Check sheet for the modelled part. Datum: model origin and axes. Units: mm. Face numbers are marked on the shaded views. A direction names the side the tool comes from. Round coordinates to 2 decimals unless told otherwise and drop trailing zeros. Loops run counter-clockwise (first coordinate to the right, second up) from the corner with the lowest first, then second, coordinate; pieces in that order, holes last. Notation, with made-up numbers: (81.25, -8.5) - (125.25, -8.5) arc R21 cw to (125.25, 19.5) - close; hole circle Ø8 at (13.25, 35.5). An arc over 180 degrees is marked (long way). Answer in a Markdown table with one row per item. Add a question column.
(1) Access from +Z, -Z, +X, -X, +Y, -Y to the whole of each face (thin tool, end or side, straight path). Record for the marked faces 1, 2, 3 and 4.
(2) Thickness scan on line 1 along Y through (x, z) = (0, 3.75); line 2 along Y through (x, z) = (2.5, 1.6); line 3 along Y through (x, z) = (-3, 2.25). Record the ranges inside material, lowest first.
(3) Gauge pin test, flat ends, axial feed: pin 1 (1.9 mm diameter, centred on x = 0, y = -8, fed in from -Z); pin 2 (1.8 mm diameter, centred on x = 1, y = -6.5, fed in from -Z); pin 3 (2.5 mm diameter, centred on x = 3.5, y = 0, fed in from +Z). Record the tip position at first contact, or that the pin passes through.
(4) Cross-section at A-A on z = 4.65. Enter the section's corners in (x, y).
(5) Cross-section at C-C on z = 3.1. Enter the section's corners in (x, y).
(6) Mould release check, pull along X, two halves, no side actions. Record for the marked faces 5, 6 and 7: +X half, -X half, draft (parallel to the pull), parting line (faces both ways), or undercut.
(7) Cross-section at B-B on x = 0. Enter the section's corners in (y, z), then the cut area to 3 significant figures.
(8) Cross-section at D-D on y = 0.5. Enter the section's corners in (x, z).
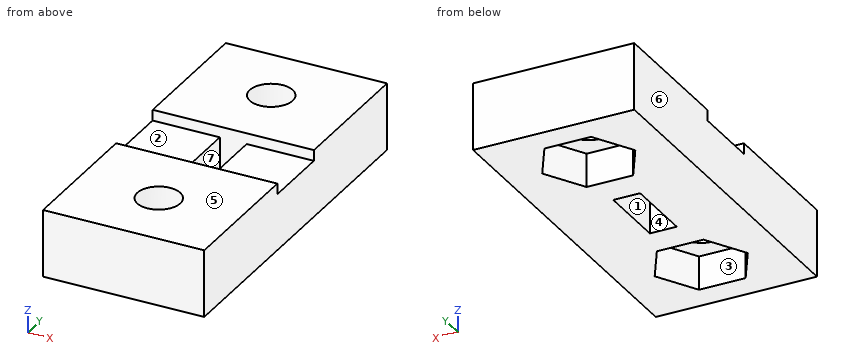
from build123d import *

# Parameters (mm, degrees)
SKETCH1_W           = 12
SKETCH1_H           = 26
SKETCH1_R           = 1.6
SKETCH1_W_2         = 2
SKETCH1_H_2         = 5.2
BOSS_EXTRUDE1_DEPTH = 5
SKETCH3_W           = 12
SKETCH3_H           = 5.2
CUT_EXTRUDE1_DEPTH  = 0.8
CUT_EXTRUDE2_DEPTH  = 2.5


with BuildPart() as part:
    # Sketch1 → Boss-Extrude1 (new body)
    with BuildSketch(Plane.XY):
        Rectangle(SKETCH1_W, SKETCH1_H)
        with Locations((0, 8)):
            Circle(SKETCH1_R, mode=Mode.SUBTRACT)
        with Locations((0, -8)):
            Circle(SKETCH1_R, mode=Mode.SUBTRACT)
        Rectangle(SKETCH1_W_2, SKETCH1_H_2, mode=Mode.SUBTRACT)
    extrude(amount=BOSS_EXTRUDE1_DEPTH)

    # Sketch3 → Cut-Extrude1 (cut)
    with BuildSketch(Plane.XY.offset(5)):
        Rectangle(SKETCH3_W, SKETCH3_H)
    extrude(amount=-CUT_EXTRUDE1_DEPTH, mode=Mode.SUBTRACT)

    # Sketch4 → Cut-Extrude2 (cut)
    with BuildSketch(Plane(origin=(0, 0, 0), x_dir=(-1, 0, 0), z_dir=(0, 0, -1))):
        Polygon((1.732050808, 11), (-1.732050808, 11), (-3.464101615, 8), (-1.732050808, 5), (1.732050808, 5), (3.464101615, 8), align=None)
        Polygon((1.732050808, -5), (-1.732050808, -5), (-3.464101615, -8), (-1.732050808, -11), (1.732050808, -11), (3.464101615, -8), align=None)
    extrude(amount=-CUT_EXTRUDE2_DEPTH, mode=Mode.SUBTRACT)


solid = part.part
Answers:
| question | item | result |
|---|---|---|
| 1 | face 1 | +Z, -Z |
| 1 | face 2 | +Z, +X, -X |
| 1 | face 3 | -Z |
| 1 | face 4 | +Z |
| 2 | line 1 | y = -13 to -9.6, -6.4 to -2.6, 2.6 to 6.4, 9.6 to 13 |
| 2 | line 2 | y = -13 to -9.67, -6.33 to 6.33, 9.67 to 13 |
| 2 | line 3 | y = -13 to -8.8, -7.2 to 7.2, 8.8 to 13 |
| 3 | pin 1 | passes through |
| 3 | pin 2 | stops at z = 2.5 |
| 3 | pin 3 | stops at z = 4.2 |
| 4 | outline | (-6, -13) - (6, -13) - (6, -2.6) - (-6, -2.6) - close; (-6, 2.6) - (6, 2.6) - (6, 13) - (-6, 13) - close; hole circle Ø3.2 at (0, -8); hole circle Ø3.2 at (0, 8) |
| 5 | outline | (-6, -13) - (6, -13) - (6, 13) - (-6, 13) - close; hole circle Ø3.2 at (0, -8); hole circle Ø3.2 at (0, 8); hole (-1, -2.6) - (1, -2.6) - (1, 2.6) - (-1, 2.6) - close |
| 6 | face 5 | draft |
| 6 | face 6 | -X half |
| 6 | face 7 | undercut |
| 7 | outline | (-13, 0) - (-11, 0) - (-11, 2.5) - (-9.6, 2.5) - (-9.6, 5) - (-13, 5) - close; (-6.4, 2.5) - (-5, 2.5) - (-5, 0) - (-2.6, 0) - (-2.6, 5) - (-6.4, 5) - close; (2.6, 0) - (5, 0) - (5, 2.5) - (6.4, 2.5) - (6.4, 5) - (2.6, 5) - close; (9.6, 2.5) - (11, 2.5) - (11, 0) - (13, 0) - (13, 5) - (9.6, 5) - close |
| 7 | area | 58.0 mm^2 |
| 8 | outline | (-6, 0) - (-1, 0) - (-1, 4.2) - (-6, 4.2) - close; (1, 0) - (6, 0) - (6, 4.2) - (1, 4.2) - close |
